```python
from build123d import *

# Parameters (mm, degrees)
BOSS_EXTRUDE1_DEPTH = 6.35
CAVITY1_START       = -6.35
CAVITY1_OUTLINE_R   = 12.7
CAVITY1_DEPTH       = 12.7


# Read off the part's stored shape, not the designer's step: Cavity1
with BuildPart() as part:
    # Sketch1 → Boss-Extrude1 (new, symmetric)
    with BuildSketch(Plane.XY):
        Polygon((-215.9, 0), (215.9, 0), (215.9, 25.4), (241.3, 25.4), (241.3, 101.6), (-241.3, 101.6), (-241.3, 25.4), (-215.9, 25.4), align=None)
    extrude(amount=BOSS_EXTRUDE1_DEPTH, both=True)

    # Cavity1 outline → Cavity1 (cut)
    with BuildSketch(Plane.XY.offset(CAVITY1_START)):
        with Locations((50.8, 51.5)):
            Circle(CAVITY1_OUTLINE_R)
    extrude(amount=CAVITY1_DEPTH, mode=Mode.SUBTRACT)


solid = part.part
```
Source: CAD feature listing. Evaluate the final solid. Frame: model axes, mm. A direction names the side the tool comes from. Give positions to 0.01 mm unless a question says otherwise; leave off trailing zeros. Order: outer loops, then holes, each group sorted by start corner. A loop starts at its lowest first (then second) coordinate and runs counter-clockwise, first axis right, second up.
(1) Material intervals for line 1 along Y through (x, z) = (50.8, 3.25); line 2 along X through (y, z) = (50, -4.25); line 3 along X through (y, z) = (7, -0.25), sorted ascending.
(2) Section query A-A (y = 51.5). Return the cut outline in (x, z).
(3) Pull-direction query (X, two-part tool) for faces 1 (the face through (228, 25.4, 0)), 2 (the face through (38.112, 52.058, -0.089)), 3 (the face through (-241.3, 64, 0)); classes: +X half, -X half, draft (parallel to the pull), parting line (faces both ways), or undercut.
(4) Section query B-B (x = 50.8). Return the cut outline in (y, z), plus the area to 3 significant figures.
(5) Access query for faces 4 (the face through (-3, 52, 6.35)), 5 (the face through (-215.9, 13, 0)), 6 (the face through (215.9, 13, 0)). Directions: +Z, -Z, +X, -X, +Y, -Y. A direction counts if a zero-diameter tool reaches every point of the face in a straight line with its end or side. Return the directions, or none.
(6) Section query C-C (z = -2). Return the cut outline in (x, y).
(7) Contact query for flat-ended pins moving along their axis: P1, Ø15, axis at x = 50.8, y = 51.5, coming from the -Z side; P2, Ø4, axis at y = 10, z = 3, coming from the -X side. Output: stop coordinate, or through.
Outcome:
1. line 1: y = 0 to 38.8, 64.2 to 101.6
1. line 2: x = -241.3 to 38.19, 63.41 to 241.3
1. line 3: x = -215.9 to 215.9
2. outline: (-241.3, -6.35) - (38.1, -6.35) - (38.1, 6.35) - (-241.3, 6.35) - close; (63.5, -6.35) - (241.3, -6.35) - (241.3, 6.35) - (63.5, 6.35) - close
3. face 1: draft
3. face 2: undercut
3. face 3: -X half
4. outline: (0, -6.35) - (38.8, -6.35) - (38.8, 6.35) - (0, 6.35) - close; (64.2, -6.35) - (101.6, -6.35) - (101.6, 6.35) - (64.2, 6.35) - close
4. area: 968 mm2
5. face 4: +Z, +X, -X, +Y, -Y
5. face 5: +Z, -Z, -X, -Y
5. face 6: +Z, -Z, +X, -Y
6. outline: (-241.3, 25.4) - (-215.9, 25.4) - (-215.9, 0) - (215.9, 0) - (215.9, 25.4) - (241.3, 25.4) - (241.3, 101.6) - (-241.3, 101.6) - close; hole circle Ø25.4 at (50.8, 51.5)
7. P1: passes through
7. P2: stops at x = -215.9
